Source: CAD feature listing. Evaluate the final solid. Frame: model axes, mm. Coordinates: 2 decimals unless noted, no trailing zeros. Loops run counter-clockwise (first coordinate to the right, second up) from the corner with the lowest first, then second, coordinate; pieces in that order, holes last. Notation, with made-up numbers: M 78,-13 L 99,-13 A28 cw 99,25 Z; hole C 80,-22.5 d7. An arc over 180 degrees is marked long. Write each question's results on one line, items separated by ' | '. Start each with the question number.
from build123d import *

# Parameters (mm, degrees)
SKETCH1_R           = 3
BOSS_EXTRUDE1_DEPTH = 200
CUT_EXTRUDE1_DEPTH  = 201
M3_TAPPED_HOLE1_D   = 2.5
M3_TAPPED_HOLE2_D   = 2.5
CUT_EXTRUDE2_START  = -1.2
SKETCH9_R           = 3
SKETCH9_R_2         = 2.5
CUT_EXTRUDE2_DEPTH  = 0.8


with BuildPart() as part:
    # Sketch1 → Boss-Extrude1 (new body)
    with BuildSketch(Plane.XY):
        Circle(SKETCH1_R)
    extrude(amount=BOSS_EXTRUDE1_DEPTH)

    # Sketch2 → Cut-Extrude1 (cut, through all)
    with BuildSketch(Plane.XY.offset(200)):
        with BuildLine():
            Line((-1.658312395, 2.5), (1.658312395, 2.5))
            ThreePointArc((1.658312395, 2.5), (0, 3), (-1.658312395, 2.5))
        make_face()
    extrude(amount=-CUT_EXTRUDE1_DEPTH, mode=Mode.SUBTRACT)

    # M3 Tapped Hole1 (through all)
    with Locations(Plane(origin=(0, 2.5, 167.7), x_dir=(0, 0, 1), z_dir=(0, 1, 0))):
        with Locations((0, 0), (-15, 0), (-120.4, 0), (-135.4, 0)):
            Hole(M3_TAPPED_HOLE1_D / 2)

    # M3 Tapped Hole2 (through all)
    with Locations(Plane(origin=(0, 2.5, 64.548836503), x_dir=(0, 0, 1), z_dir=(0, 1, 0))):
        with Locations((0, 0)):
            Hole(M3_TAPPED_HOLE2_D / 2)

    # Sketch9 → Cut-Extrude2 (cut)
    with BuildSketch(Plane.XY.offset(200).offset(CUT_EXTRUDE2_START)):
        Circle(SKETCH9_R)
        Circle(SKETCH9_R_2, mode=Mode.SUBTRACT)
    cut_extrude2 = extrude(amount=-CUT_EXTRUDE2_DEPTH, mode=Mode.SUBTRACT)

    # Mirror1: Cut-Extrude2 across plane
    add(cut_extrude2.mirror(Plane.XY.offset(100)), mode=Mode.SUBTRACT)


solid = part.part
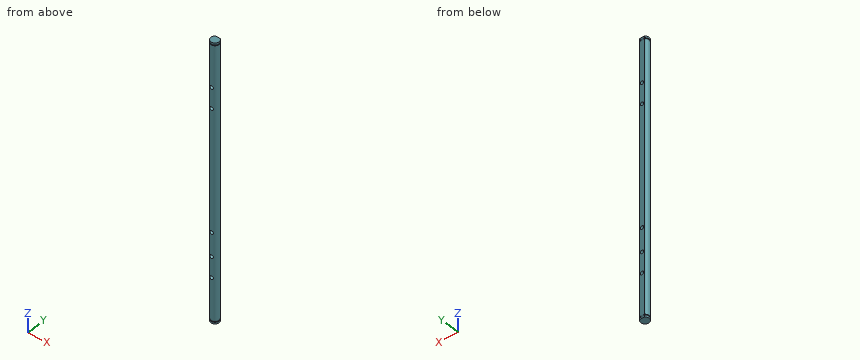
Item 1: Cut plane A-A (y = 0). Output: boundary loops of the cut face in (x, z).
Item 2: Cut plane B-B (z = 52). Output: boundary loops of the cut face in (x, y), then the cut area to 3 significant figures.
Item 3: Line query: probe 1 along Z at (x, y) = (0, 0.7); probe 2 along Z at (x, y) = (2.75, 0.5); probe 3 along Z at (x, y) = (-1, -0.35). Output: solid intervals per line, ascending.
Item 4: First-contact query: pin 1 Ø1.5 at (x, z) = (0, 32.3) entering from -Y; pin 2 Ø2 at (y, z) = (1.5, 51) entering from -X. Flat tips, straight axial feed; report the tip coordinate or a pass-through.
Response values:
1) outline: M -3,0 L 3,0 L 3,1.2 L 2.5,1.2 L 2.5,2 L 3,2 L 3,198 L 2.5,198 L 2.5,198.8 L 3,198.8 L 3,200 L -3,200 L -3,198.8 L -2.5,198.8 L -2.5,198 L -3,198 L -3,2 L -2.5,2 L -2.5,1.2 L -3,1.2 Z; hole C 0,32.3 d2.5; hole C 0,47.3 d2.5; hole C 0,64.55 d2.5; hole C 0,152.7 d2.5; hole C 0,167.7 d2.5
2) outline: M -1.66,2.5 A3 ccw long 1.66,2.5 Z | area: 27.1 mm2
3) probe 1: z = 0 to 31.05, 33.55 to 46.05, 48.55 to 63.3, 65.8 to 151.45, 153.95 to 166.45, 168.95 to 200 | probe 2: z = 0 to 1.2, 2 to 198, 198.8 to 200 | probe 3: z = 0 to 31.55, 33.05 to 46.55, 48.05 to 63.8, 65.3 to 151.95, 153.45 to 166.95, 168.45 to 200
4) pin 1: passes through | pin 2: stops at x = -2.96
